from build123d import *

# Parameters (mm, degrees)
F0_R     = 27
F1_DEPTH = 2


with BuildPart() as f1:
    # F0 (on Front) → F1 (new body)
    with BuildSketch(Plane.XZ):
        Circle(F0_R)
        with BuildLine():
            ThreePointArc((23.776413, 7.725425), (24.692209, 3.910862), (25, 0))
            ThreePointArc((25, 0), (24.692209, -3.910862), (23.776413, -7.725425))
            ThreePointArc((23.776413, -7.725425), (22.275163, -11.349762), (20.225425, -14.694631))
            ThreePointArc((20.225425, -14.694631), (17.67767, -17.67767), (14.694631, -20.225425))
            ThreePointArc((14.694631, -20.225425), (11.349762, -22.275163), (7.725425, -23.776413))
            ThreePointArc((7.725425, -23.776413), (3.910862, -24.692209), (0, -25))
            ThreePointArc((0, -25), (-3.910862, -24.692209), (-7.725425, -23.776413))
            ThreePointArc((-7.725425, -23.776413), (-11.349762, -22.275163), (-14.694631, -20.225425))
            ThreePointArc((-14.694631, -20.225425), (-17.67767, -17.67767), (-20.225425, -14.694631))
            ThreePointArc((-20.225425, -14.694631), (-22.275163, -11.349762), (-23.776413, -7.725425))
            ThreePointArc((-23.776413, -7.725425), (-24.692209, -3.910862), (-25, 0))
            ThreePointArc((-25, 0), (-24.692209, 3.910862), (-23.776413, 7.725425))
            ThreePointArc((-23.776413, 7.725425), (-22.275163, 11.349762), (-20.225425, 14.694631))
            ThreePointArc((-20.225425, 14.694631), (-17.67767, 17.67767), (-14.694631, 20.225425))
            ThreePointArc((-14.694631, 20.225425), (-11.349762, 22.275163), (-7.725425, 23.776413))
            ThreePointArc((-7.725425, 23.776413), (-3.910862, 24.692209), (0, 25))
            ThreePointArc((0, 25), (3.910862, 24.692209), (7.725425, 23.776413))
            ThreePointArc((7.725425, 23.776413), (11.349762, 22.275163), (14.694631, 20.225425))
            ThreePointArc((14.694631, 20.225425), (17.67767, 17.67767), (20.225425, 14.694631))
            ThreePointArc((20.225425, 14.694631), (22.275163, 11.349762), (23.776413, 7.725425))
        make_face(mode=Mode.SUBTRACT)
    extrude(amount=F1_DEPTH)


solid = f1.part
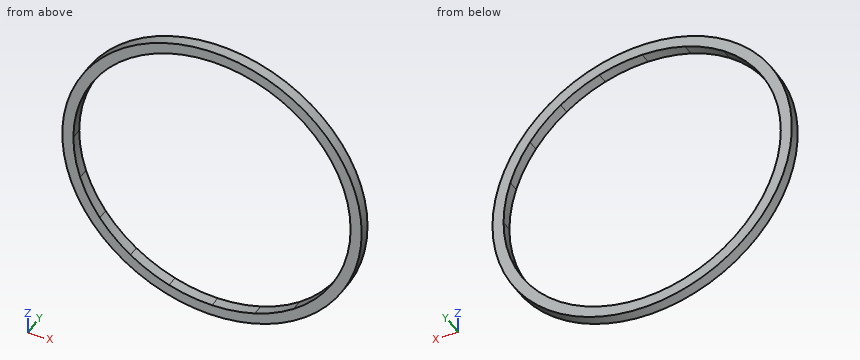
Check sheet for the modelled part. Datum: model origin and axes. Units: mm. Give positions to 0.01 mm unless a question says otherwise; leave off trailing zeros. Order: outer loops, then holes, each group sorted by start corner. A loop starts at its lowest first (then second) coordinate and runs counter-clockwise, first axis right, second up. Notation, with made-up numbers: M 89.25,43.5 L 112.25,43.5 A13 ccw 112.25,54.5 Z; hole C 86.5,39 d7. An arc over 180 degrees is marked long. Answer as CSV lines item,"result". Start each with the question number.
Item 1: Cross-section at C-C on x = -5. Enter the section's corners in (y, z).
Item 2: Gauge pin test, flat ends, axial feed: P1, Ø1, axis at x = 4, y = -1, coming from the +Z side; P2, Ø1, axis at x = -13, y = 0, coming from the +Z side; P3, Ø1, axis at x = -11.5, y = -1.5, coming from the -Z side. Record the tip position at first contact, or that the pin passes through.
Item 3: Cross-section at B-B on z = 3. Enter the section's corners in (x, y), plus the area to 3 significant figures.
Item 4: Cross-section at A-A on y = -0.6. Enter the section's corners in (x, z), plus the area to 3 significant figures.
Item 5: Thickness scan on line 1 (Z direction, x = 0.5, y = -1.1) (3 decimals); line 2 (Z direction, x = -7, y = -1.75); line 3 (X direction, y = -1.25, z = -22). Record the ranges inside material, lowest first. Write a range as [from, to].
Established:
1,outline,"M -2,-26.53 L 0,-26.53 L 0,-24.49 L -2,-24.49 Z; M -2,24.49 L 0,24.49 L 0,26.53 L -2,26.53 Z"
2,P1,"stops at z = 26.77"
2,P2,"stops at z = 23.93"
2,P3,"stops at z = -24.66"
3,outline,"M -26.83,-2 L -24.82,-2 L -24.82,0 L -26.83,0 Z; M 24.82,-2 L 26.83,-2 L 26.83,0 L 24.82,0 Z"
3,area,"8.05 mm^2"
4,outline,"C 0,0 d54; hole M -25,0 A25 ccw -23.78,-7.73 A25 ccw -20.23,-14.69 A25 ccw -14.69,-20.23 A25 ccw -7.73,-23.78 A25 ccw 0,-25 A25 ccw 7.73,-23.78 A25 ccw 14.69,-20.23 A25 ccw 20.23,-14.69 A25 ccw 23.78,-7.73 A25 ccw 25,0 A25 ccw 23.78,7.73 A25 ccw 20.23,14.69 A25 ccw 14.69,20.23 A25 ccw 7.73,23.78 A25 ccw 0,25 A25 ccw -7.73,23.78 A25 ccw -14.69,20.23 A25 ccw -20.23,14.69 A25 ccw -23.78,7.73 A25 ccw Z"
4,area,"327 mm^2"
5,line 1,"z = [-26.995, -24.995], [24.995, 26.995]"
5,line 2,"z = [-26.08, -24], [24, 26.08]"
5,line 3,"x = [-15.65, -11.87], [11.87, 15.65]"
